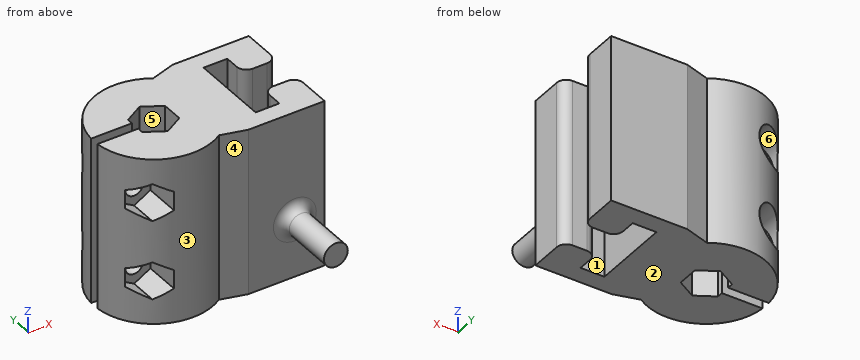
from build123d import *

# Parameters (mm, degrees)
BOSS_EXTRUDE1_DEPTH = 35
SKETCH2_R           = 1.8669
CUT_EXTRUDE1_DEPTH  = 45.791182168
SKETCH3_R           = 3.9497
CUT_EXTRUDE2_DEPTH  = 8
CUT_EXTRUDE3_DEPTH  = 8
BOSS_EXTRUDE2_DEPTH = 35
FILLET1_R           = 2
SKETCH6_R           = 2.5
BOSS_EXTRUDE3_DEPTH = 13
FILLET2_R           = 2


with BuildPart() as part:
    # Sketch1 → Boss-Extrude1 (new body)
    with BuildSketch(Plane.XY):
        with BuildLine():
            ThreePointArc((12.5, 0), (0.500401124, 12.489979933), (-12.459935794, 1))
            Line((-12.459935794, 1), (-3.9, 1))
            Line((-3.9, 1), (-3.9, 2.25166605))
            Line((-3.9, 2.25166605), (0, 4.5033321))
            Line((0, 4.5033321), (3.9, 2.25166605))
            Line((3.9, 2.25166605), (3.9, -2.25166605))
            Line((3.9, -2.25166605), (0, -4.5033321))
            Line((0, -4.5033321), (-3.9, -2.25166605))
            Line((-3.9, -2.25166605), (-3.9, -1))
            Line((-3.9, -1), (-12.459935794, -1))
            ThreePointArc((-12.459935794, -1), (0.500401124, -12.489979933), (12.5, 0))
        make_face()
    extrude(amount=BOSS_EXTRUDE1_DEPTH)

    # Sketch2 → Cut-Extrude1 (cut, through all)
    with BuildSketch(Plane(origin=(0, 12.5, 0), x_dir=(1, 0, 0), z_dir=(0, 1, 0))):
        with Locations(Location((-7.078786681, -9.175485886, 0), (0, 0, 270))):
            Circle(SKETCH2_R)
        with Locations(Location((-7.078786681, -25.824514114, 0), (0, 0, 270))):
            Circle(SKETCH2_R)
    extrude(amount=-CUT_EXTRUDE1_DEPTH, mode=Mode.SUBTRACT)

    # Sketch3 → Cut-Extrude2 (cut)
    with BuildSketch(Plane(origin=(0, 12.5, 0), x_dir=(1, 0, 0), z_dir=(0, 1, 0))):
        with Locations(Location((-7.078786681, -9.175485886, 0), (0, 0, 270))):
            Circle(SKETCH3_R)
        with Locations(Location((-7.078786681, -25.824514114, 0), (0, 0, 270))):
            Circle(SKETCH3_R)
    extrude(amount=-CUT_EXTRUDE2_DEPTH, mode=Mode.SUBTRACT)

    # Sketch4 → Cut-Extrude3 (cut)
    with BuildSketch(Plane(origin=(0, -12.5, 0), x_dir=(-1, 0, 0), z_dir=(0, -1, 0))):
        Polygon((7.078786681, -5.230682437), (3.662486681, -7.203084162), (3.662486681, -11.147887611), (7.078786681, -13.120289335), (10.495086681, -11.147887611), (10.495086681, -7.203084162), align=None)
        Polygon((7.078786681, -21.879710665), (3.662486681, -23.852112389), (3.662486681, -27.796915838), (7.078786681, -29.769317563), (10.495086681, -27.796915838), (10.495086681, -23.852112389), align=None)
    extrude(amount=-CUT_EXTRUDE3_DEPTH, mode=Mode.SUBTRACT)

    # Sketch5 → Boss-Extrude2 (add, through all)
    with BuildSketch(Plane(origin=(0, 0, 0), x_dir=(-1, 0, 0), z_dir=(0, 0, -1))):
        with BuildLine():
            Line((-12, 12.083333333), (-6.827937157, 10.470399905))
            ThreePointArc((-6.827937157, 10.470399905), (-12.499949552, -0.035513444), (-6.768332777, -10.509028091))
            Line((-6.768332777, -10.509028091), (-12, -11.916666667))
            Line((-12, -11.916666667), (-28, -11.916666667))
            Line((-28, -11.916666667), (-28, -3.166666667))
            Line((-28, -3.166666667), (-21, -3.166666667))
            Line((-21, -3.166666667), (-21, -8.166666667))
            Line((-21, -8.166666667), (-16, -8.166666667))
            Line((-16, -8.166666667), (-16, 8.333333333))
            Line((-16, 8.333333333), (-21, 8.333333333))
            Line((-21, 8.333333333), (-21, 3.333333333))
            Line((-21, 3.333333333), (-28, 3.333333333))
            Line((-28, 3.333333333), (-28, 12.083333333))
            Line((-28, 12.083333333), (-12, 12.083333333))
        make_face()
    extrude(amount=-BOSS_EXTRUDE2_DEPTH)

    # Fillet1
    fillet1_edges = [part.edges().sort_by_distance(p)[0] for p in [
        (28, -3.166666667, 17.5),
        (21, -3.166666667, 17.5),
        (21, 3.333333333, 17.5),
        (28, 3.333333333, 17.5),
    ]]
    fillet(fillet1_edges, radius=FILLET1_R)

    # Sketch6 → Boss-Extrude3 (add)
    with BuildSketch(Plane.XZ.offset(11.916666667)):
        with Locations(Location((21.762676708, 12.114369006, 0), (0, 0, 90))):
            Circle(SKETCH6_R)
    extrude(amount=BOSS_EXTRUDE3_DEPTH)

    # Fillet2
    fillet2_edges = [part.edges().sort_by_distance(p)[0] for p in [
        (21.762676708, -11.916666667, 9.614369006),
    ]]
    fillet(fillet2_edges, radius=FILLET2_R)


solid = part.part
Geometry check sheet. Reference: the model listing, model coordinates, mm. Face numbers are marked on the shaded views. A direction names the side the tool comes from. Give positions to 0.01 mm unless a question says otherwise; leave off trailing zeros. Loops run counter-clockwise (first coordinate to the right, second up) from the corner with the lowest first, then second, coordinate; pieces in that order, holes last. Notation, with made-up numbers: M 59,67.25 L 92,67.25 A34 cw 92,103.25 Z; hole C -34,54.25 d6. An arc over 180 degrees is marked long. Answer as a JSON object with one key per item and string values. Group by question number.
Item 1: Sectioned sample at A-A on z = 18. Record the boundary of the cut face in (x, y).
Item 2: Sectioned sample at D-D on z = 27. Give the number of separate pieces and of enclosed holes in the cut face, plus the area to 3 significant figures.
Item 3: Sectioned sample at C-C on y = -9.5. Record the boundary of the cut face in (x, z), plus the area to 3 significant figures.
Item 4: Gauge pin test, flat ends, axial feed: pin 1 (12.5 mm diameter, centred on x = -7.08, z = 25.82, fed in from +Y); pin 2 (2.5 mm diameter, centred on x = 18.5, z = 25, fed in from +Y); pin 3 (3.5 mm diameter, centred on y = 6.5, z = 10.5, fed in from -X). Record the tip position at first contact, or that the pin passes through.
Item 5: Access from +Z, -Z, +X, -X, +Y, -Y to the whole of each face (thin tool, end or side, straight path). Record for the marked faces 4, 5 and 6.
Item 6: Sectioned sample at B-B on x = 2. Record the boundary of the cut face in (y, z).
Item 7: Mould release check, pull along Y, two halves, no side actions. Record for the marked faces 1, 2 and 3: pulls with the +Y half, pulls with the -Y half, needs draft (parallel to the pull), parting line crosses it, or undercut.
Item 8: Material ranges on L1, parallel to Y at x = 25.5, z = 20; L2, parallel to Y at x = 20, z = 4.5; L3, parallel to X at y = 2.5, z = 9, recorded low to high.
Findings below:
{
 "1": {"outline": "M -12.46,-1 A12.5 ccw 6.77,-10.51 L 12,-11.92 L 28,-11.92 L 28,-5.17 A2 ccw 26,-3.17 L 23,-3.17 A2 ccw 21,-5.17 L 21,-8.17 L 16,-8.17 L 16,8.33 L 21,8.33 L 21,5.33 A2 ccw 23,3.33 L 26,3.33 A2 ccw 28,5.33 L 28,12.08 L 12,12.08 L 6.83,10.47 A12.5 ccw -12.46,1 L -3.9,1 L -3.9,2.25 L 0,4.5 L 3.9,2.25 L 3.9,-2.25 L 0,-4.5 L -3.9,-2.25 L -3.9,-1 Z"},
 "2": {"separate pieces": "3", "enclosed holes": "0", "area": "607 mm2"},
 "3": {"outline": "M -8.12,0 L 28,0 L 28,35 L -8.12,35 L -8.12,29.17 L -7.08,29.77 L -3.66,27.8 L -3.66,23.85 L -7.08,21.88 L -8.12,22.48 L -8.12,12.52 L -7.08,13.12 L -3.66,11.15 L -3.66,7.2 L -7.08,5.23 L -8.12,5.83 Z", "area": "1,210 mm2"},
 "4": {"pin 1": "y = 12.47", "pin 2": "y = 12.08", "pin 3": "x = -11.56"},
 "5": {"face 4": "+Z, -Z, -Y", "face 5": "+Z, -Z", "face 6": "+Y"},
 "6": {"outline": "M -12.34,0 L -3.35,0 L -3.35,35 L -12.34,35 Z; M 3.35,0 L 12.34,0 L 12.34,35 L 3.35,35 Z"},
 "7": {"face 1": "undercut", "face 2": "needs draft", "face 3": "pulls with the -Y half"},
 "8": {"L1": "-11.92 to -3.17, 3.33 to 12.08", "L2": "-11.92 to -8.17, 8.33 to 12.08", "L3": "-12.25 to -8.94, -5.22 to -3.47, 3.47 to 16"}
}
